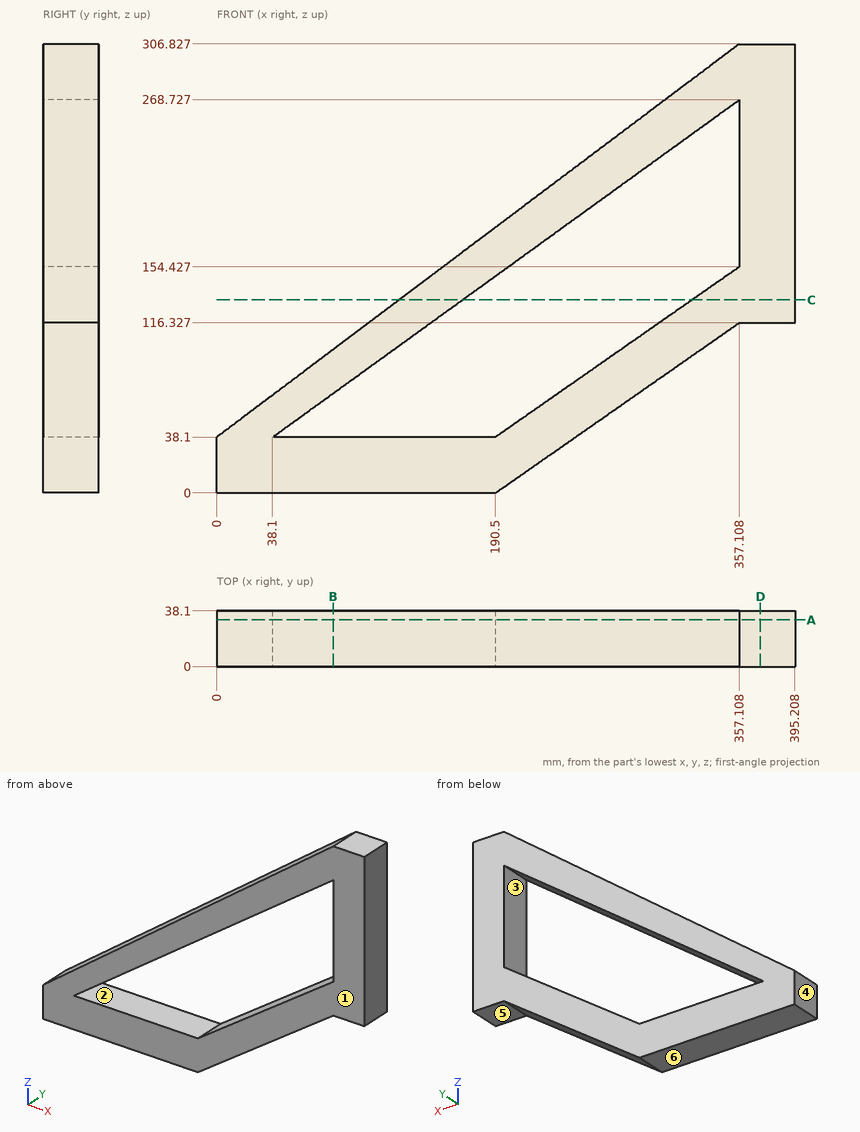
Verification items for this drawing (mm, ordinates from the low corner). A direction names the side the tool comes from. Coordinates: 2 decimals unless noted, no trailing zeros. Write each loop counter-clockwise with the first axis right and the second up, starting at its lowest first coordinate (ties: lowest second). Pieces come first, ordered by that corner, then holes. Notation, with made-up numbers: M 32.25,89.5 L 79.25,89.5 A8 ccw 79.25,99.5 Z; hole C 6,60.5 d5. An arc over 180 degrees is marked long. One line per item, written item: value. Start each with the question number.
(1) Scan lines: line 1 along X through (y, z) = (36, 97); line 2 along X through (y, z) = (3.5, 241.5) (1 decimal); line 3 along Z through (x, y) = (57.5, 3.5) (1 decimal). Record each from-to range of solid material in increasing order. Write a range as [from, to].
(2) Tool access check on the marked faces 5 and 6. Record the directions out of +Z, -Z, +X, -X, +Y, -Y that give a thin tool (end or side, any length) a straight path to the whole face; none if there is none.
(3) Sectioned sample at D-D, the plane x = 371.5. Enter the section's corners in (y, z).
(4) Sectioned sample at C-C, the plane z = 132. Enter the section's corners in (x, y) (1 decimal).
(5) Sectioned sample at A-A, the plane y = 32. Enter the section's corners in (x, z).
(6) Release check for a two-part mould opening along X. For the marked faces 1, 2, 3 and 4 record: released by +X, released by -X, zero draft, split by the parting line, or undercut.
(7) Sectioned sample at B-B, the plane x = 79.5. Enter the section's corners in (y, z).
(8) Depth check by flat-ended pin: pin 1 (3 mm diameter, centred on x = 290.5, y = 20, fed in from -Z); pin 2 (1.5 mm diameter, centred on x = 47, y = 29.5, fed in from +Z); pin 3 (19 mm diameter, centred on x = 373.5, y = 18.5, fed in from -Z). Enter the tip coordinate at first touch or a pass-through.
Filled sheet:
1. line 1: [78.27, 119.57], [274.86, 329.43]
1. line 2: [270.3, 319.4], [357.1, 395.2]
1. line 3: [0, 38.1], [52.1, 81.4]
2. face 5: -Z, +X, +Y, -Y
2. face 6: -Z, +X, -X, +Y, -Y
3. outline: M 0,116.33 L 38.1,116.33 L 38.1,306.83 L 0,306.83 Z
4. outline: M 124.8,0 L 168,0 L 168,38.1 L 124.8,38.1 Z; M 325,0 L 395.2,0 L 395.2,38.1 L 325,38.1 Z
5. outline: M 0,0 L 190.5,0 L 357.11,116.33 L 395.21,116.33 L 395.21,306.83 L 357.11,306.83 L 0,38.1 Z; hole M 38.1,38.1 L 190.5,38.1 L 357.11,154.43 L 357.11,268.73 Z
6. face 1: zero draft
6. face 2: undercut
6. face 3: undercut
6. face 4: released by -X
7. outline: M 0,0 L 38.1,0 L 38.1,38.1 L 0,38.1 Z; M 0,68.03 L 38.1,68.03 L 38.1,97.92 L 0,97.92 Z
8. pin 1: z = 68.77
8. pin 2: z = 74.03
8. pin 3: z = 116.33
